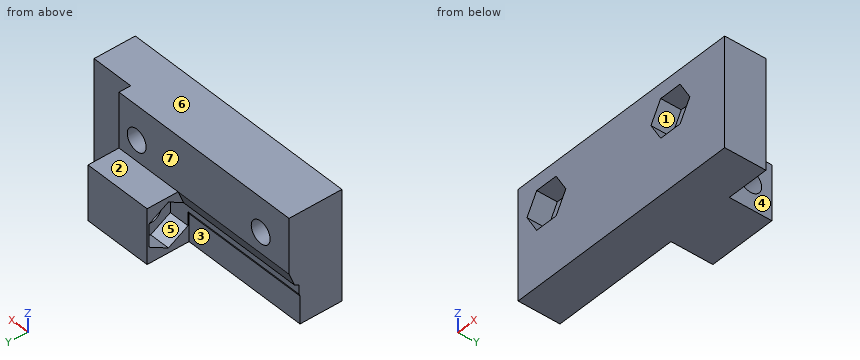
from build123d import *

# Parameters (mm, degrees)
SALIENTE_EXTRUIR1_DEPTH           = 8
SALIENTE_EXTRUIR2_DEPTH           = 8
CORTAR_EXTRUIR1_REACH             = 30.8
CROQUIS3_R                        = 1.6
CORTAR_EXTRUIR2_REACH             = 9.7
CROQUIS4_R                        = 1.6
CORTAR_EXTRUIR3_DEPTH             = 3
CORTAR_EXTRUIR4_DEPTH             = 18.8
CORTAR_EXTRUIR5_DEPTH             = 3
CORTAR_EXTRUIR5_DIRECTION_2_REACH = 20.8


with BuildPart() as part:
    # Croquis1 → Saliente-Extruir1 (new body)
    with BuildSketch(Plane.XY):
        Polygon((0, 0), (0, 6), (-6.2, 6), (-6.2, 12.2), (-35, 12.2), (-35, 0), align=None)
    extrude(amount=SALIENTE_EXTRUIR1_DEPTH)

    # Croquis2 → Saliente-Extruir2 (add)
    with BuildSketch(Plane.XY.offset(8)):
        Polygon((-6.2, 7.7), (-35, 7.7), (-35, 0), (0, 0), (0, 6), (-6.2, 6), align=None)
    extrude(amount=SALIENTE_EXTRUIR2_DEPTH)

    # Croquis3 → Cortar-Extruir1 (cut, up to next)
    with BuildSketch(Plane(origin=(-6.2, 0, 0), x_dir=(0, 0, -1), z_dir=(1, 0, 0)), mode=Mode.PRIVATE) as cortar_extruir1_sk1:
        with Locations((-4, 9.1)):
            Circle(CROQUIS3_R)
    cortar_extruir1_tool1 = extrude(cortar_extruir1_sk1.sketch, amount=-CORTAR_EXTRUIR1_REACH, mode=Mode.PRIVATE) & part.part
    add(cortar_extruir1_tool1.solids().sort_by_distance((-6.2, 9.1, 4))[0], mode=Mode.SUBTRACT)

    # Croquis4 → Cortar-Extruir2 (cut, up to next)
    with BuildSketch(Plane(origin=(0, 7.7, 0), x_dir=(1, 0, 0), z_dir=(0, 1, 0)), mode=Mode.PRIVATE) as cortar_extruir2_sk1:
        with Locations((-30.2, -11)):
            Circle(CROQUIS4_R)
    cortar_extruir2_tool1 = extrude(cortar_extruir2_sk1.sketch, amount=-CORTAR_EXTRUIR2_REACH, mode=Mode.PRIVATE) & part.part
    add(cortar_extruir2_tool1.solids().sort_by_distance((-30.2, 7.7, 11))[0], mode=Mode.SUBTRACT)
    # Croquis4 → Cortar-Extruir2 (cut, up to next)
    with BuildSketch(Plane(origin=(0, 7.7, 0), x_dir=(1, 0, 0), z_dir=(0, 1, 0)), mode=Mode.PRIVATE) as cortar_extruir2_sk2:
        with Locations((-9.2, -11)):
            Circle(CROQUIS4_R)
    cortar_extruir2_tool2 = extrude(cortar_extruir2_sk2.sketch, amount=-CORTAR_EXTRUIR2_REACH, mode=Mode.PRIVATE) & part.part
    add(cortar_extruir2_tool2.solids().sort_by_distance((-9.2, 7.7, 11))[0], mode=Mode.SUBTRACT)

    # Croquis5 → Cortar-Extruir3 (cut)
    with BuildSketch(Plane.XZ):
        Polygon((-33.490896534, 11), (-31.845448267, 8.15), (-28.554551733, 8.15), (-26.909103466, 11), (-28.554551733, 13.85), (-31.845448267, 13.85), align=None)
        Polygon((-12.490896534, 11), (-10.845448267, 8.15), (-7.554551733, 8.15), (-5.909103466, 11), (-7.554551733, 13.85), (-10.845448267, 13.85), align=None)
    extrude(amount=-CORTAR_EXTRUIR3_DEPTH, mode=Mode.SUBTRACT)

    # Croquis6 → Cortar-Extruir4 (cut)
    with BuildSketch(Plane.ZY.offset(35)):
        Polygon((8, 7.7), (4, 6.1), (0, 6.1), (0, 12.2), (8, 12.2), align=None)
    extrude(amount=-CORTAR_EXTRUIR4_DEPTH, mode=Mode.SUBTRACT)

    # Croquis7 → Cortar-Extruir5 (cut)
    with BuildSketch(Plane.ZY.offset(16.2)):
        Polygon((0.709103466, 9.1), (2.354551733, 6.25), (5.645448267, 6.25), (7.290896534, 9.1), (5.645448267, 11.95), (2.354551733, 11.95), align=None)
    extrude(amount=-CORTAR_EXTRUIR5_DEPTH, mode=Mode.SUBTRACT)

    # Croquis7 → Cortar-Extruir5 direction 2 (cut, up to next)
    with BuildSketch(Plane.ZY.offset(16.2), mode=Mode.PRIVATE) as cortar_extruir5_direction_2_sk1:
        Polygon((0.709103466, 9.1), (2.354551733, 6.25), (5.645448267, 6.25), (7.290896534, 9.1), (5.645448267, 11.95), (2.354551733, 11.95), align=None)
    cortar_extruir5_direction_2_tool1 = extrude(cortar_extruir5_direction_2_sk1.sketch, amount=CORTAR_EXTRUIR5_DIRECTION_2_REACH, mode=Mode.PRIVATE) & part.part
    add(cortar_extruir5_direction_2_tool1.solids().sort_by_distance((-16.2, 9.1, 4))[0], mode=Mode.SUBTRACT)


solid = part.part
Part model, mm, in its own coordinate system. Face numbers are marked on the shaded views. A direction names the side the tool comes from. Give positions to 0.01 mm unless a question says otherwise; leave off trailing zeros. Write each loop counter-clockwise with the first axis right and the second up, starting at its lowest first coordinate (ties: lowest second). Pieces come first, ordered by that corner, then holes.
1) Pin check, flat tips, straight feed: pin 1 (3 mm diameter, centred on x = -26.5, z = 2, fed in from +Y); pin 2 (3.5 mm diameter, centred on x = -10.5, y = 9.5, fed in from +Z); pin 3 (1.9 mm diameter, centred on x = -4, z = 11.5, fed in from +Y). Stop position of each tip, or through.
Resolved:
pin 1: stops at y = 6.1
pin 2: stops at z = 8
pin 3: stops at y = 6
2) Two-plate mould, pull along Z, no slides. Class the marked faces 5, 6 and 7: released by +Z, released by -Z, zero draft, split by the parting line, or undercut.
Resolved:
face 5: undercut
face 6: released by +Z
face 7: zero draft
3) Cut at D-D on y = 1.25. Write the cut outline in (x, z), then the cut area to 3 significant figures.
Resolved:
outline: (-35, 0) - (0, 0) - (0, 16) - (-35, 16) - close; hole (-33.49, 11) - (-31.85, 8.15) - (-28.55, 8.15) - (-26.91, 11) - (-28.55, 13.85) - (-31.85, 13.85) - close; hole (-12.49, 11) - (-10.85, 8.15) - (-7.55, 8.15) - (-5.91, 11) - (-7.55, 13.85) - (-10.85, 13.85) - close
area: 504 mm2
4) Cut at A-A on x = -9.2. Write the cut outline in (y, z), then the cut area to 3 significant figures.
Resolved:
outline: (0, 0) - (12.2, 0) - (12.2, 8) - (7.7, 8) - (7.7, 9.4) - (3, 9.4) - (3, 8.15) - (0, 8.15) - close; (0, 13.85) - (3, 13.85) - (3, 12.6) - (7.7, 12.6) - (7.7, 16) - (0, 16) - close; hole circle Ø3.2 at (9.1, 4)
area: 119 mm2
5) Probe L1, parallel to X at y = 6.25, z = 11; L2, parallel to X at y = 5.9, z = 11; L3, parallel to Y at x = -8.25, z = 4. List the from-to ranges inside material, lowest first.
Resolved:
L1: x = -35 to -31.8, -28.6 to -10.8, -7.6 to -6.2
L2: x = -35 to -31.8, -28.6 to -10.8, -7.6 to 0
L3: y = 0 to 7.5, 10.7 to 12.2
6) Cut at B-B on x = -30.2. Write the cut outline in (y, z) (3 decimals).
Resolved:
outline: (0, 0) - (6.1, 0) - (6.1, 4) - (6.25, 4.375) - (6.25, 5.645) - (6.911, 6.027) - (7.7, 8) - (7.7, 9.4) - (3, 9.4) - (3, 8.15) - (0, 8.15) - close; (0, 13.85) - (3, 13.85) - (3, 12.6) - (7.7, 12.6) - (7.7, 16) - (0, 16) - close
7) Which spindle directions (+Z, -Z, +X, -X, +Y, -Y) get a long thin tool onto all of the face, cutting with end or side? Do the marked faces 1, 2, 3 and 4. Say none if no direction does.
Resolved:
face 1: -Y
face 2: +Z, +X, -X, +Y
face 3: -Z, -X, +Y
face 4: +Z, -Z, +X, +Y
8) Cut at C-C on z = 9.75. Write the cut outline in (x, y), then the cut area to 3 significant figures.
Resolved:
outline: (-35, 0) - (-32.77, 0) - (-32.77, 3) - (-31.2, 3) - (-31.2, 7.7) - (-35, 7.7) - close; (-29.2, 3) - (-27.63, 3) - (-27.63, 0) - (-11.77, 0) - (-11.77, 3) - (-10.2, 3) - (-10.2, 7.7) - (-29.2, 7.7) - close; (-8.2, 3) - (-6.63, 3) - (-6.63, 0) - (0, 0) - (0, 6) - (-6.2, 6) - (-6.2, 7.7) - (-8.2, 7.7) - close
area: 209 mm2
